Read the model definition and answer for the solid it produces. Units are mm, in the model's axes. A direction names the side the tool comes from. Give positions to 0.01 mm unless a question says otherwise; leave off trailing zeros. Order: outer loops, then holes, each group sorted by start corner. A loop starts at its lowest first (then second) coordinate and runs counter-clockwise, first axis right, second up. Notation, with made-up numbers: (22.25, 28.25) -> (33.25, 28.25) arc R23 cw to (33.25, 66.25) -> close; hole circle Ø11 at (69.5, -20). An arc over 180 degrees is marked (long way). Answer as CSV lines item,"result". Start each with the question number.
1) The mould has two halves that part along Y. Classify faces 1 (the face through (-27.436, 49, -23)), 2 (the face through (-17, 26.853, 9)), 3 (the face through (-41, 67.493, -12)), 4 (the face through (-17, -135.707, -32)): +Y half, -Y half, draft (parallel to the pull), parting line (faces both ways), or undercut.
2) Flat-ended cylindrical pins translate along their axes: pin 1 Ø20.5 at (x, z) = (-47.5, -8) entering from -Y; pin 2 Ø4 at (y, z) = (43.5, -21.5) entering from +X; pin 3 Ø8 at (y, z) = (-22.5, 0.5) entering from -X. Find the tip coordinate at first contact, or state that the pin passes through.
3) For faces 5 (the face through (-42, 47, 0)), 6 (the face through (-45.358, 51.082, -20.527)), 7 (the face through (-17.1, 25.33, -26.85)), 8 (the face through (-17.098, 25.405, 1.528)), 9 (the face through (-33, 49, -5.08)), determine the directions among +Z, -Z, +X, -X, +Y, -Y from which every point of the face is accessible in a straight line to the end or side of a thin tool.
4) Find section C-C (y = 35). Determine the outline of the cut face in (x, z).
5) Find section B-B (z = 8.5). Determine the outline of the cut face in (x, y).
6) Find section A-A (y = -110). Determine the outline of the cut face in (x, z), and give its area (3 significant figures).
7) Find section D-D (z = -8). Determine the outline of the cut face in (x, y), and give its area (3 significant figures).
8) Straight lines are drawn through the part: L1, parallel to Z at x = -28.5, y = -119; L2, parallel to Z at x = -34, y = 54; L3, parallel to X at y = 55, z = 8.5. For each, find the intervals that lie inside material, in ascending order. Write a range as from..to.
```python
from build123d import *

# Parameters (mm, degrees)
BASE_EXTRUDE_DEPTH  = 25.4
SKETCH7_W           = 12.7
SKETCH7_H           = 38.1
BOSS_EXTRUDE5_DEPTH = 25.4
SKETCH8_W           = 25.751736715
SKETCH8_H           = 31.75
CUT_EXTRUDE5_DEPTH  = 25.4
SKETCH11_W          = 12.7
SKETCH11_H          = 40.64
BOSS_EXTRUDE6_DEPTH = 25.4
SKETCH12_W          = 25.4
SKETCH12_H          = 38.1
CUT_EXTRUDE7_DEPTH  = 22.86
SKETCH13_R          = 7.62
CUT_EXTRUDE8_DEPTH  = 20.32
CUT_EXTRUDE9_START  = -50.8
SKETCH14_R          = 7.62
CUT_EXTRUDE9_DEPTH  = 50.8
CUT_EXTRUDE10_REACH = 216.029
SKETCH15_W          = 20.32
SKETCH15_H          = 15.24
FILLET1_R           = 5.08


with BuildPart() as part:
    # Sketch1 → Base-Extrude (new body)
    with BuildSketch(Plane.XY):
        Polygon((-4.57611336, -135.706612686), (-29.97611336, -135.706612686), (-29.97611336, 26.853387314), (-55.37611336, 26.853387314), (-55.37611336, 67.493387314), (-29.97611336, 67.493387314), (-4.57611336, 67.493387314), align=None)
    extrude(amount=-BASE_EXTRUDE_DEPTH)

    # Sketch7 → Boss-Extrude5 (add)
    with BuildSketch(Plane.ZY.offset(29.97611336)):
        with Locations((-31.75, -116.656612686)):
            Rectangle(SKETCH7_W, SKETCH7_H)
        with Locations((6.35, -116.656612686)):
            Rectangle(SKETCH7_W, SKETCH7_H)
    extrude(amount=-BOSS_EXTRUDE5_DEPTH)

    # Sketch8 → Cut-Extrude5 (cut)
    with BuildSketch(Plane.ZY.offset(29.97611336)):
        with Locations((-12.524131643, -119.831612686)):
            Rectangle(SKETCH8_W, SKETCH8_H)
    extrude(amount=-CUT_EXTRUDE5_DEPTH, mode=Mode.SUBTRACT)

    # Sketch11 → Boss-Extrude6 (add)
    with BuildSketch(Plane(origin=(-4.57611336, 0, 0), x_dir=(0, 0, -1), z_dir=(1, 0, 0))):
        with Locations((31.75, 47.173387314)):
            Rectangle(SKETCH11_W, SKETCH11_H)
        with Locations((-6.35, 47.173387314)):
            Rectangle(SKETCH11_W, SKETCH11_H)
    extrude(amount=-BOSS_EXTRUDE6_DEPTH)

    # Sketch12 → Cut-Extrude7 (cut)
    with BuildSketch(Plane(origin=(-4.57611336, 0, 0), x_dir=(0, 0, -1), z_dir=(1, 0, 0))):
        with Locations((12.7, 48.443387314)):
            Rectangle(SKETCH12_W, SKETCH12_H)
    extrude(amount=-CUT_EXTRUDE7_DEPTH, mode=Mode.SUBTRACT)

    # Sketch13 → Cut-Extrude8 (cut)
    with BuildSketch(Plane.ZY.offset(55.37611336)):
        with Locations(Location((-13.088541232, 49.429752215, 0), (0, 0, 270))):
            Circle(SKETCH13_R)
    extrude(amount=-CUT_EXTRUDE8_DEPTH, mode=Mode.SUBTRACT)

    # Sketch14 → Cut-Extrude9 (cut)
    with BuildSketch(Plane(origin=(0, 0, -38.1), x_dir=(-1, 0, 0), z_dir=(0, 0, -1)).offset(CUT_EXTRUDE9_START)):
        with Locations(Location((16.00611336, 54.793387314, 0), (0, 0, 90))):
            Circle(SKETCH14_R)
        with Locations(Location((17.931310165, -123.006612686, 0), (0, 0, 90))):
            Circle(SKETCH14_R)
    extrude(amount=CUT_EXTRUDE9_DEPTH, mode=Mode.SUBTRACT)

    # Cut-Extrude10: up to this face of the body (flat: up to its plane)
    cut_extrude10_end = Plane(part.part.faces().sort_by_distance((-16.00611336, 29.393387314, -12.7))[0])
    # Sketch15 → Cut-Extrude10 (cut, up to the picked face)
    with BuildSketch(Plane(origin=(0, 67.493387314, 0), x_dir=(1, 0, 0), z_dir=(0, 1, 0)), mode=Mode.PRIVATE) as cut_extrude10_sk1:
        with Locations((-27.43611336, 12.7)):
            Rectangle(SKETCH15_W, SKETCH15_H)
    cut_extrude10_tool1 = split(extrude(cut_extrude10_sk1.sketch, amount=-CUT_EXTRUDE10_REACH, mode=Mode.PRIVATE), bisect_by=cut_extrude10_end, keep=Keep.BOTH, mode=Mode.PRIVATE)
    add(cut_extrude10_tool1.solids().sort_by(Axis((-27.436113, 67.493387, -12.7), (0, -1, 0)))[0], mode=Mode.SUBTRACT)

    # Fillet1
    # the kernel refuses this fillet: 5.08 mm, written as the material it adds along each edge
    with BuildSketch(Plane(origin=(-29.97611336, -97.606612686, 0), x_dir=(0, 1, 0), z_dir=(1, 0, 0)), Plane(origin=(-29.97611336, -97.606612686, -25.4), x_dir=(0, 0, -1), z_dir=(1, 0, 0)), Plane(origin=(-4.57611336, 26.853387314, 0), x_dir=(0, -1, 0), z_dir=(-1, 0, 0))) as fillet1_piece_1:
        with BuildLine():
            CenterArc((FILLET1_R, FILLET1_R), FILLET1_R, 180, 90)
            Line((0, FILLET1_R), (0, 0))
            Line((0, 0), (FILLET1_R, 0))
        make_face()
    extrude(amount=25.4)
    with BuildSketch(Plane(origin=(-4.57611336, 26.853387314, -25.4), x_dir=(0, -1, 0), z_dir=(-1, 0, 0))) as fillet1_piece_2:
        with BuildLine():
            CenterArc((FILLET1_R, -FILLET1_R), FILLET1_R, 90, 90)
            Line((0, -FILLET1_R), (0, 0))
            Line((0, 0), (FILLET1_R, 0))
        make_face()
    extrude(amount=25.4)


solid = part.part
```
Findings below:
1,face 1,"draft"
1,face 2,"undercut"
1,face 3,"+Y half"
1,face 4,"-Y half"
2,pin 1,"y = 26.85"
2,pin 2,"x = -27.44"
2,pin 3,"x = -29.98"
3,face 5,"+Z, -X, +Y, -Y"
3,face 6,"-X"
3,face 7,"-Z, +X, -X"
3,face 8,"+Z, +X, -X"
3,face 9,"+X, +Y"
4,outline,"(-55.38, -25.4) -> (-29.98, -25.4) -> (-29.98, -38.1) -> (-4.58, -38.1) -> (-4.58, -25.4) -> (-27.44, -25.4) -> (-27.44, -20.32) -> (-37.6, -20.32) -> (-37.6, -5.08) -> (-27.44, -5.08) -> (-27.44, 0) -> (-4.58, 0) -> (-4.58, 12.7) -> (-29.98, 12.7) -> (-29.98, 0) -> (-55.38, 0) -> close"
5,outline,"(-29.98, -135.71) -> (-4.58, -135.71) -> (-4.58, -97.61) -> (-29.98, -97.61) -> close; (-29.98, 26.85) -> (-4.58, 26.85) -> (-4.58, 67.49) -> (-29.98, 67.49) -> close; hole circle Ø15.24 at (-17.93, -123.01); hole circle Ø15.24 at (-16.01, 54.79)"
6,outline,"(-29.98, -38.1) -> (-4.58, -38.1) -> (-4.58, -25.4) -> (-29.98, -25.4) -> close; (-29.98, 0.35) -> (-4.58, 0.35) -> (-4.58, 12.7) -> (-29.98, 12.7) -> close"
6,area,"636 mm²"
7,outline,"(-55.38, 26.85) -> (-29.98, 26.85) -> (-29.98, -103.96) -> (-4.58, -103.96) -> (-4.58, 29.39) -> (-37.6, 29.39) -> (-37.6, 43.76) -> (-55.38, 43.76) -> close; (-55.38, 55.1) -> (-37.6, 55.1) -> (-37.6, 67.49) -> (-55.38, 67.49) -> close"
7,area,"3,930 mm²"
8,L1,"-38.1..-25.4, 0.35..12.7"
8,L2,"-25.4..-20.32, -5.08..0"
8,L3,"-29.98..-23.62, -8.39..-4.58"
